Geometry check sheet. Reference: drawing and pictorial views, mm from the part's lowest x, y, z. Round coordinates to 2 decimals unless told otherwise and drop trailing zeros. Write each loop counter-clockwise with the first axis right and the second up, starting at its lowest first coordinate (ties: lowest second). Pieces come first, ordered by that corner, then holes. Notation, with made-up numbers: M 85,84.25 L 104,84.25 A34 ccw 104,114.25 Z; hole C 69,-6.5 d2. An arc over 180 degrees is marked long. Put each result on its own line as item: value. Start each with the question number.
(1) Material ranges on probe 1 along Z at (x, y) = (0.75, 176.5); probe 2 along Y at (x, z) = (3.25, 35); probe 3 along Y at (x, z) = (0.5, 48), recorded low to high.
(2) Section check B-B on y = 166.5. Record the cut outline in (x, z).
(3) Gauge pin test, flat end, axial feed: pin 1 (1.9 mm diameter, centred on x = 2, y = 155, fed in from +Z). Record the tip position at first contact, or that the pin passes through.
(4) Section check D-D on z = 15.5. Record the cut outline in (x, y), then the cut area to 3 significant figures.
(5) Section check C-C on x = 1.75. Count the separate pieces of the cut face and the enclosed holes in it, then the cut area to 3 significant figures.
(6) Section check A-A on z = 51. Record the cut outline in (x, y), then the cut area to 3 significant figures.
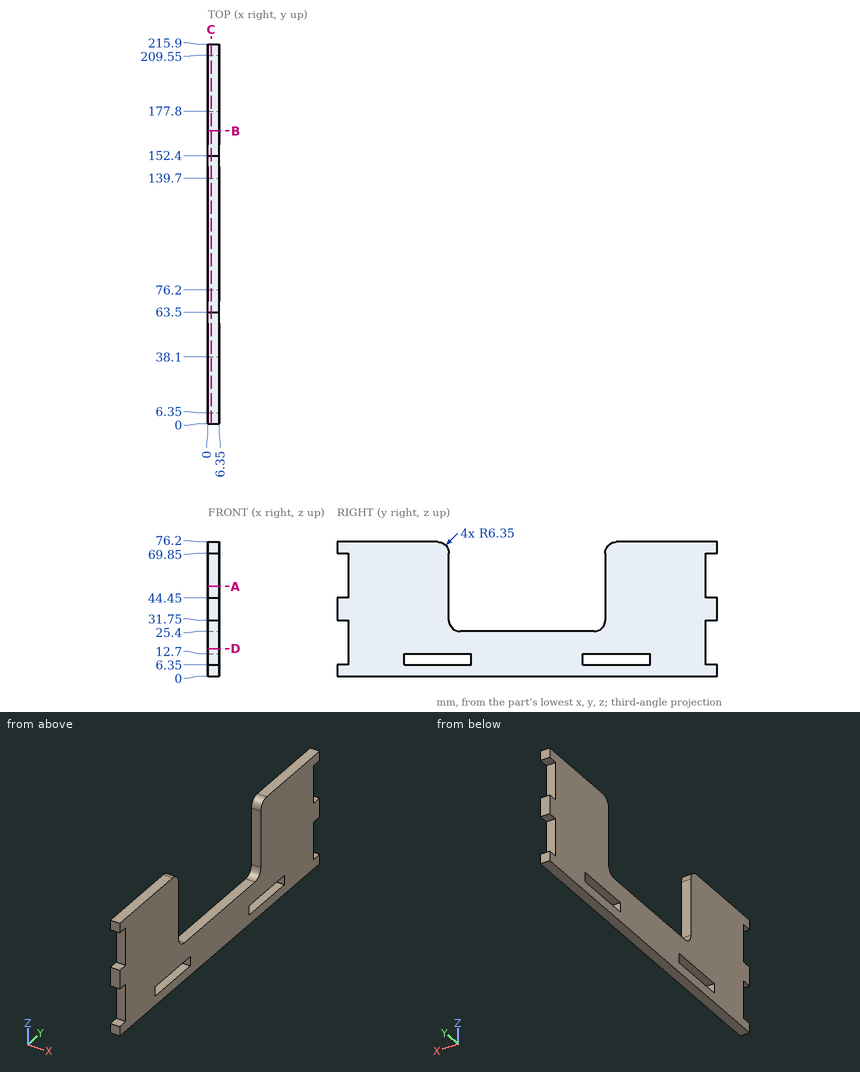
Answers follow:
1. probe 1: z = 0 to 6.35, 12.7 to 76.2
1. probe 2: y = 0 to 63.5, 152.4 to 215.9
1. probe 3: y = 6.35 to 63.5, 152.4 to 209.55
2. outline: M 0,0 L 6.35,0 L 6.35,6.35 L 0,6.35 Z; M 0,12.7 L 6.35,12.7 L 6.35,76.2 L 0,76.2 Z
3. pin 1: stops at z = 75.55
4. outline: M 0,6.35 L 6.35,6.35 L 6.35,209.55 L 0,209.55 Z
4. area: 1,290 mm^2
5. separate pieces: 1
5. enclosed holes: 2
5. area: 10,800 mm^2
6. outline: M 0,6.35 L 6.35,6.35 L 6.35,63.5 L 0,63.5 Z; M 0,152.4 L 6.35,152.4 L 6.35,209.55 L 0,209.55 Z
6. area: 726 mm^2
